The model under review builds one solid part; all positions refer to its coordinate system, in mm. A direction names the side the tool comes from. Round coordinates to 2 decimals unless told otherwise and drop trailing zeros. Write each loop counter-clockwise with the first axis right and the second up, starting at its lowest first coordinate (ties: lowest second). Pieces come first, ordered by that corner, then holes. Notation, with made-up numbers: (-11, 14) -> (47, 14) arc R26 ccw to (47, 38) -> close; hole circle Ø7 at (35, 38.25). An arc over 180 degrees is marked (long way). Answer as a JSON object with one key per item and string values. Group by question number.
1) To check wall thickness, follow probe 1 along Y at (x, z) = (0, -21.1); probe 2 along Y at (x, z) = (0, 3.6); probe 3 along Y at (x, z) = (4.25, -5.25). State the ranges of each line that lie inside material, in increasing order. Write a range as [from, to].
2) Machinability: for faces 1 (the flat face through (0, 29, -25)), 2 (the flat face through (-5, 0, 0)), 3 (the flat face through (0, 15, -7)), which of the approach directions +Z, -Z, +X, -X, +Y, -Y give a long, thin tool a straight path to every point of the face, cutting with its end or side? Answer none if there is none.
3) We need section B-B, the plane x = 0. Write out the cut boundary in (y, z).
4) We need section C-C, the plane x = -5.5. Write out the cut boundary in (y, z).
5) We need section D-D, the plane y = -0.5. Write out the cut boundary in (x, z).
6) We need section A-A, the plane y = 25. Write out the cut boundary in (x, z).
7) Mouldability with a two-part tool opening along Y and no side actions: class faces 4 (the flat face through (0, 10, -12)), 5 (the flat face through (-0.1, 4.5, 5)), 6 (the cylindrical face through (-0.417, 28.173, -22.465)), 7 (the cylindrical face through (-0.59, 3.96, 2.46)) as pulls with the +Y half, pulls with the -Y half, needs draft (parallel to the pull), parting line crosses it, or undercut.
8) Insertion check: pin 1 Ø1.5 at (y, z) = (9, -10.5) entering from -X; pin 2 Ø5 at (x, z) = (-4.5, -20.5) entering from -Y. Each pin has a flat end and moves straight along its axis. Give the tip position at first contact, or say it passes through.
from build123d import *

# Parameters (mm, degrees)
SKETCH1_R           = 4.5
BOSS_EXTRUDE1_DEPTH = 5
SKETCH2_W           = 20
SKETCH2_H           = 39
BOSS_EXTRUDE2_DEPTH = 25
CUT_EXTRUDE1_DEPTH  = 30
SKETCH4_R           = 3.2
CUT_EXTRUDE2_DEPTH  = 10
FILLET1_R           = 2
FILLET2_R           = 1
SKETCH5_W           = 20
SKETCH5_H           = 9
CUT_EXTRUDE3_DEPTH  = 10
FILLET3_R           = 2


with BuildPart() as part:
    # Sketch1 → Boss-Extrude1 (new body)
    with BuildSketch(Plane.XY):
        Polygon((-10, 10), (-10, -10), (-10, -11), (10, -11), (10, -10), (10, 10), (10, 44), (-10, 44), align=None)
        with Locations((0, -0.5)):
            Circle(SKETCH1_R, mode=Mode.SUBTRACT)
    extrude(amount=BOSS_EXTRUDE1_DEPTH)

    # Sketch2 → Boss-Extrude2 (add)
    with BuildSketch(Plane(origin=(0, 0, 0), x_dir=(-1, 0, 0), z_dir=(0, 0, -1))):
        with Locations((0, 29.5)):
            Rectangle(SKETCH2_W, SKETCH2_H)
    extrude(amount=BOSS_EXTRUDE2_DEPTH)

    # Sketch3 → Cut-Extrude1 (cut)
    with BuildSketch(Plane(origin=(10, 0, 0), x_dir=(0, 0, -1), z_dir=(1, 0, 0))):
        Polygon((0, 15), (-5, 15), (-5, 49), (20, 49), (20, 15), align=None)
    extrude(amount=-CUT_EXTRUDE1_DEPTH, mode=Mode.SUBTRACT)

    # Sketch4 → Cut-Extrude2 (cut)
    with BuildSketch(Plane.XY.offset(-20)):
        with Locations((0, 25)):
            Circle(SKETCH4_R)
    extrude(amount=-CUT_EXTRUDE2_DEPTH, mode=Mode.SUBTRACT)

    # Fillet1
    fillet1_edges = [part.edges().sort_by_distance(p)[0] for p in [
        (0, 15, -20),
    ]]
    fillet(fillet1_edges, radius=FILLET1_R)

    # Fillet2
    fillet2_edges = [part.edges().sort_by_distance(p)[0] for p in [
        (0, 15, 5),
    ]]
    fillet(fillet2_edges, radius=FILLET2_R)

    # Sketch5 → Cut-Extrude3 (cut)
    with BuildSketch(Plane.XY.offset(-20)):
        with Locations((0, 44.5)):
            Rectangle(SKETCH5_W, SKETCH5_H)
    extrude(amount=-CUT_EXTRUDE3_DEPTH, mode=Mode.SUBTRACT)

    # Fillet3
    fillet3_edges = [part.edges().sort_by_distance(p)[0] for p in [
        (10, 40, -22.5),
        (-10, 40, -22.5),
    ]]
    fillet(fillet3_edges, radius=FILLET3_R)


solid = part.part
Here are the results:
{
 "1": {"probe 1": "y = [10, 21.8], [28.2, 40]", "probe 2": "y = [-11, -5], [4, 15]", "probe 3": "y = [10, 15]"},
 "2": {"face 1": "-Z, +X, -X, +Y, -Y", "face 2": "-Z, +X, -X, -Y", "face 3": "+Z, +X, -X, +Y"},
 "3": {"outline": "(-11, 0) -> (-5, 0) -> (-5, 5) -> (-11, 5) -> close; (4, 0) -> (10, 0) -> (10, -25) -> (21.8, -25) -> (21.8, -20) -> (17, -20) arc R2 cw to (15, -18) -> (15, 4) arc R1 ccw to (14, 5) -> (4, 5) -> close; (28.2, -25) -> (40, -25) -> (40, -20) -> (28.2, -20) -> close"},
 "4": {"outline": "(-11, 0) -> (10, 0) -> (10, -25) -> (40, -25) -> (40, -20) -> (17, -20) arc R2 cw to (15, -18) -> (15, 4) arc R1 ccw to (14, 5) -> (-11, 5) -> close"},
 "5": {"outline": "(-10, 0) -> (-4.5, 0) -> (-4.5, 5) -> (-10, 5) -> close; (4.5, 0) -> (10, 0) -> (10, 5) -> (4.5, 5) -> close"},
 "6": {"outline": "(-10, -25) -> (-3.2, -25) -> (-3.2, -20) -> (-10, -20) -> close; (3.2, -25) -> (10, -25) -> (10, -20) -> (3.2, -20) -> close"},
 "7": {"face 4": "pulls with the -Y half", "face 5": "needs draft", "face 6": "undercut", "face 7": "undercut"},
 "8": {"pin 1": "passes through", "pin 2": "stops at y = 10"}
}
